Check sheet for the modelled part. Datum: model origin and axes. Units: mm. A direction names the side the tool comes from. Round coordinates to 2 decimals unless told otherwise and drop trailing zeros. Write each loop counter-clockwise with the first axis right and the second up, starting at its lowest first coordinate (ties: lowest second). Pieces come first, ordered by that corner, then holes. Notation, with made-up numbers: (47.25, -32.5) - (70.25, -32.5) arc R19 cw to (70.25, -5.5) - close; hole circle Ø1 at (-31.75, -15.75). An arc over 180 degrees is marked (long way). Answer as a JSON object with one key per item and string values. Group by question number.
Item 1: Sectioned sample at C-C on x = 110. Record the boundary of the cut face in (y, z).
Item 2: Release check for a two-part mould opening along Y. For faces 6 (the flat face through (77, 23, 2.6)), 7 (the flat face through (3, 33.625, 13)), 8 (the flat face through (1.5, 23.5, 20.1)) record: pulls with the +Y half, pulls with the -Y half, needs draft (parallel to the pull), parting line crosses it, or undercut.
Item 3: Sectioned sample at D-D on y = 9.5. Record the boundary of the cut face in (x, z).
Item 4: Sectioned sample at A-A on z = 9. Record the boundary of the cut face in (x, y) (3 decimals).
Item 5: Gauge pin test, flat ends, axial feed: P1, Ø5, axis at x = 150, z = 9.5, coming from the -Y side (3 decimals); P2, Ø9, axis at y = 27, z = 12, coming from the +X side; P3, Ø0.6, axis at x = 0.5, y = 24, coming from the -Z side; P4, Ø8, axis at y = 7.5, z = 13.5, coming from the -X side. Record the tip position at first contact, or that the pin passes through.
Item 6: Set-up check for faces 1 (the flat face through (150.727, 24, 7)), 2 (the flat face through (149, 13.625, 13)), 3 (the flat face through (65, 43, 5.2)), 4 (the flat face through (1.727, 23, 7)), 5 (the flat face through (77, 4.65, 4)): record each of +Z, -Z, +X, -X, +Y, -Y from which the full face is reachable in a straight line by a thin tool's end or side.
Item 7: Thickness scan on line 1 (Y direction, x = 139, z = 2.75); line 2 (X direction, y = 25, z = 14); line 3 (Z direction, x = 40, y = 28.5). Record the ranges inside material, lowest first.
Autodesk Fusion 360 part; units mm, degrees
sketch "Base" plane through (0, 0, 0) normal (0, 0, 1) x (1, 0, 0)
  line L0 (1.7267, 45) -> (150.7267, 45)
  line L1 (150.7267, 45) -> (150.7267, 2.25)
  line L2 (150.7267, 2.25) -> (1.7267, 2.25)
  line L3 (1.7267, 2.25) -> (1.7267, 45)
  dimension "d1" = 149
  dimension "d2" = 42.75
extrude "Extrude1" add sketch "Base" along normal blind 5.2
sketch "Frame" plane through (0, 0, 5.2) normal (0, 0, 1) x (-1, 0, 0)
  line L0 (-1.7267, -2.25) -> (-150.7267, -2.25)
  line L1 (-150.7267, -2.25) -> (-150.7267, -45)
  line L2 (-150.7267, -45) -> (-1.7267, -45)
  line L3 (-1.7267, -45) -> (-1.7267, -2.25)
  line L4 (-4.3267, -42.6) -> (-148.1267, -42.6)
  line L5 (-148.1267, -42.6) -> (-148.1267, -4.65)
  line L6 (-148.1267, -4.65) -> (-4.3267, -4.65)
  line L7 (-4.3267, -4.65) -> (-4.3267, -42.6)
  dimension "d5" = 2.4
  dimension "d6" = 2.6
  dimension "d7" = 2.4
  dimension "d8" = 2.6
extrude "Extrude2" cut sketch "Frame" against normal blind 2.6 contours L4 L5 L6 L7
sketch "Hook" plane through (0, 0, 5.2) normal (0, 0, 1) x (-1, 0, 0)
  line L0 (-148.1267, -42.6) -> (-148.1267, -4.65)
  line L1 (-148.1267, -4.65) -> (-4.3267, -4.65)
  line L2 (-4.3267, -4.65) -> (-4.3267, -42.6)
  line L3 (-4.3267, -42.6) -> (-148.1267, -42.6)
  line L4 (-1.7267, -2.25) -> (-150.7267, -2.25)
  line L5 (-150.7267, -2.25) -> (-150.7267, -45)
  line L6 (-150.7267, -45) -> (-1.7267, -45)
  line L7 (-1.7267, -45) -> (-1.7267, -2.25)
  line L8 (-1.7267, -33.625) -> (-4.3267, -33.625)
  line L9 (-4.3267, -13.625) -> (-1.7267, -13.625)
  line L10 (-148.1267, -33.625) -> (-150.7267, -33.625)
  line L11 (-148.1267, -13.625) -> (-150.7267, -13.625)
  dimension "d11" = 20
  dimension "d12" = 11.375
  dimension "d13" = 12.2767
  dimension "d14" = 11.375
  dimension "d15" = 20
extrude "Extrude3" add sketch "Hook" along normal blind 16 contours L0 L5 L10 L11 | L2 L7 L8 L9
sketch "Hook Left" plane through (0, 33.625, 0) normal (0, 1, 0) x (-1, 0, 0)
  line L0 (-150.7267, 5.2) -> (-148.1267, 5.2)
  line L1 (-148.1267, 5.2) -> (-148.1267, 21.2)
  line L2 (-148.1267, 21.2) -> (-150.7267, 21.2)
  line L3 (-150.7267, 21.2) -> (-150.7267, 5.2)
  line L4 (-148.1267, 21.2) -> (-152.7767, 21.2)
  line L5 (-152.7767, 21.2) -> (-152.7767, 17.55)
  line L6 (-152.7767, 17.55) -> (-148.1267, 17.55)
  line L7 (-148.1267, 17.55) -> (-148.1267, 21.2)
  dimension "d18" = 3.65
  dimension "d19" = 4.65
extrude "Extrude4" add sketch "Hook Left" against normal blind 20 contours L3 L4 L5 L6
sketch "Hook Right" plane through (0, 33.625, 0) normal (0, 1, 0) x (-1, 0, 0)
  line L0 (-4.3267, 5.2) -> (-1.7267, 5.2)
  line L1 (-1.7267, 5.2) -> (-1.7267, 21.2)
  line L2 (-1.7267, 21.2) -> (-4.3267, 21.2)
  line L3 (-4.3267, 21.2) -> (-4.3267, 5.2)
  line L4 (-4.3267, 21.2) -> (0.3233, 21.2)
  line L5 (0.3233, 21.2) -> (0.3233, 17.55)
  line L6 (0.3233, 17.55) -> (-4.3267, 17.55)
  line L7 (-4.3267, 17.55) -> (-4.3267, 21.2)
  dimension "d22" = 3.65
  dimension "d23" = 4.65
extrude "Extrude5" add sketch "Hook Right" against normal blind 20 contours L1 L4 L5 L6
chamfer "Chamfer1" distance 3.65 distance2 2.2 2 edges at (152.7767, 23.625, 21.2) (-0.3233, 23.625, 21.2) measured on face at (152.7767, 26.9583, 19.9833) measured on face at (2.7767, 20.2917, 21.2)
Completed:
{
 "1": {"outline": "(2.25, 0) - (45, 0) - (45, 5.2) - (42.6, 5.2) - (42.6, 2.6) - (4.65, 2.6) - (4.65, 5.2) - (2.25, 5.2) - close"},
 "2": {"face 6": "undercut", "face 7": "pulls with the +Y half", "face 8": "needs draft"},
 "3": {"outline": "(1.73, 0) - (150.73, 0) - (150.73, 5.2) - (148.13, 5.2) - (148.13, 2.6) - (4.33, 2.6) - (4.33, 5.2) - (1.73, 5.2) - close"},
 "4": {"outline": "(1.727, 13.625) - (4.327, 13.625) - (4.327, 33.625) - (1.727, 33.625) - close; (148.127, 13.625) - (150.727, 13.625) - (150.727, 33.625) - (148.127, 33.625) - close"},
 "5": {"P1": "y = 13.625", "P2": "x = 150.73", "P3": "z = 17.55", "P4": "through"},
 "6": {"face 1": "-Z, +X, +Y, -Y", "face 2": "+Z, +X, -X, -Y", "face 3": "+Z, +X, -X, +Y", "face 4": "-Z, -X, +Y, -Y", "face 5": "+Z"},
 "7": {"line 1": "2.25 to 4.65, 42.6 to 45", "line 2": "1.73 to 4.33, 148.13 to 150.73", "line 3": "0 to 2.6"}
}
